from build123d import *

# Parameters (mm, degrees)
SKETCH1_R               = 20.450000000000003
BOSS_EXTRUDE1_DEPTH     = 15.875
CUT_EXTRUDE2_START      = -11.875
CUT_EXTRUDE2_DEPTH      = 11.875
M4_CLEARANCE_HOLE1_D    = 4.5
CHAMFER1_SIZE           = 4.7625
SHELL1_OUTLINE_R        = 20.45
SHELL1_DEPTH            = 10.284072775
SHELL1_2_DEPTH          = 2
BOSS_EXTRUDE2_START     = 2
BOSS_EXTRUDE2_DEPTH     = 2
CUT_EXTRUDE5_DEPTH      = 0.5
CUT_EXTRUDE7_DEPTH      = 42.774640932046694
CUT_EXTRUDE7_DEPTH_BACK = 42.774640932046694


with BuildPart() as part:
    # Sketch1 → Boss-Extrude1 (new body)
    # profile 1 of 2: a face of its own
    with BuildSketch(Plane.XY):
        with BuildLine():
            ThreePointArc((-4.449768205772106, -27.620494530122933), (-6.26579346059064, -23.208178662106004), (-9.919608253272203, -20.139609532026952))
            ThreePointArc((-9.919608253272203, -20.139609532026952), (-22.449999999999612, -2.260939e-11), (-9.919608253272486, 20.139609531981904))
            ThreePointArc((-9.919608253272486, 20.139609531981904), (-6.265793460590954, 23.208178662061), (-4.449768205772483, 27.620494530077963))
            ThreePointArc((-4.449768205772483, 27.620494530077963), (1.6339e-13, 31.449999999977553), (4.449768205772869, 27.620494530078034))
            ThreePointArc((4.449768205772869, 27.620494530078034), (6.265793460591407, 23.2081786620611), (9.919608253272981, 20.139609531982046))
            ThreePointArc((9.919608253272981, 20.139609531982046), (22.4500000000004, -2.229809e-11), (9.919608253273257, -20.13960953202682))
            ThreePointArc((9.919608253273257, -20.13960953202682), (6.265793460591725, -23.20817866210592), (4.449768205773249, -27.620494530122876))
            ThreePointArc((4.449768205773249, -27.620494530122876), (5.9636e-13, -31.450000000022463), (-4.449768205772106, -27.620494530122933))
        make_face()
        Circle(SKETCH1_R, mode=Mode.SUBTRACT)
    # profile 2 of 2: a face of its own
    with BuildSketch(Plane.XY):
        Circle(SKETCH1_R)
    extrude(amount=BOSS_EXTRUDE1_DEPTH)

    # Sketch3 → Cut-Extrude2 (cut)
    with BuildSketch(Plane.XY.offset(15.875).offset(CUT_EXTRUDE2_START)):
        with BuildLine():
            ThreePointArc((-9.919608253272486, 20.139609531981908), (2.3162e-13, 22.449999999977553), (9.919608253272981, 20.13960953198205))
            ThreePointArc((9.91960825327298, 20.139609531982046), (6.2657934605914, 23.208178662061094), (4.4497682057728625, 27.620494530078037))
            ThreePointArc((4.4497682057728625, 27.620494530078037), (1.6065e-13, 31.449999999977546), (-4.449768205772477, 27.620494530077963))
            ThreePointArc((-4.449768205772479, 27.620494530077963), (-6.265793460590951, 23.208178662061), (-9.919608253272482, 20.139609531981904))
        make_face()
        with BuildLine():
            ThreePointArc((4.449768205773246, -27.62049453012288), (6.265793460591725, -23.20817866210592), (9.919608253273257, -20.13960953202682))
            ThreePointArc((9.919608253273244, -20.139609532026824), (5.4515e-13, -22.45000000002246), (-9.919608253272205, -20.139609532026956))
            ThreePointArc((-9.9196082532722, -20.139609532026952), (-6.265793460590633, -23.208178662106), (-4.449768205772095, -27.620494530122933))
            ThreePointArc((-4.4497682057720995, -27.620494530122933), (5.9608e-13, -31.450000000022456), (4.449768205773246, -27.62049453012288))
        make_face()
    extrude(amount=CUT_EXTRUDE2_DEPTH, mode=Mode.SUBTRACT)

    # M4 Clearance Hole1 (through all)
    with Locations(Plane.XY.offset(4)):
        with Locations((0, -26.95), (0, 26.95)):
            Hole(M4_CLEARANCE_HOLE1_D / 2)

    # Chamfer1
    chamfer1_edges = [part.edges().sort_by_distance(p)[0] for p in [
        (9.91960825327299, 20.139609531982046, 15.875),
    ]]
    chamfer(chamfer1_edges, length=CHAMFER1_SIZE)

    # Shell1: read off the stored shape, not the designer's step
    # Shell1 outline → Shell1 (cut)
    with BuildSketch(Plane.XY):
        Circle(SHELL1_OUTLINE_R)
    extrude(amount=SHELL1_DEPTH, mode=Mode.SUBTRACT)

    # Shell1 2 outline → Shell1 2 (cut)
    with BuildSketch(Plane.XY):
        with BuildLine():
            ThreePointArc((9.035901505, -18.345434963), (0, -20.45), (-9.035901505, -18.345434963))
            ThreePointArc((-9.035901505, -18.345434963), (-5.656595992, -20.826114024), (-3.336769132, -24.317800965))
            ThreePointArc((-3.336769132, -24.317800965), (0, -22.7), (3.336769132, -24.317800965))
            ThreePointArc((3.336769132, -24.317800965), (5.656595992, -20.826114024), (9.035901505, -18.345434963))
        make_face()
        with BuildLine():
            ThreePointArc((-3.336769132, 24.317800965), (-5.656595992, 20.826114024), (-9.035901505, 18.345434963))
            ThreePointArc((-9.035901505, 18.345434963), (0, 20.45), (9.035901505, 18.345434963))
            ThreePointArc((9.035901505, 18.345434963), (5.656595992, 20.826114024), (3.336769132, 24.317800965))
            ThreePointArc((3.336769132, 24.317800965), (0, 22.7), (-3.336769132, 24.317800965))
        make_face()
    extrude(amount=SHELL1_2_DEPTH, mode=Mode.SUBTRACT)

    # Shell1 3 outline → Shell1 3 (revolve, cut)
    with BuildSketch(Plane.XZ):
        Polygon((16.859072875, 13.875), (0, 13.875), (0, 10.284072775), (20.45, 10.284072775), align=None)
    revolve(axis=Axis((0, 0, 0), (0, 0, 1)), mode=Mode.SUBTRACT)

    # Sketch6 → Boss-Extrude2 (add)
    with BuildSketch(Plane(origin=(0, 0, 2), x_dir=(-1, 0, 0), z_dir=(0, 0, -1)).offset(BOSS_EXTRUDE2_START)):
        with BuildLine():
            ThreePointArc((9.035901504651038, -18.34543496347422), (5.656595991725949, -20.826114024149227), (3.3367691319005477, -24.3178009648972))
            ThreePointArc((3.3367691319005477, -24.3178009648972), (-5.6684e-13, -22.70000000000008), (-3.3367691319011485, -24.317800964898304))
            ThreePointArc((-3.3367691319011485, -24.317800964898304), (-5.656595991726578, -20.826114024149597), (-9.035901504652076, -18.345434963474087))
            ThreePointArc((-9.035901504652076, -18.345434963474087), (-5.3382e-13, -20.45000000002246), (9.035901504651038, -18.34543496347422))
        make_face()
        with BuildLine():
            ThreePointArc((-9.035901504651829, 18.345434963429298), (-5.65659599172108, 20.826114024110222), (-3.336769131894781, 24.31780096486728))
            ThreePointArc((-3.336769131894781, 24.31780096486728), (-2.2525e-13, 22.699999999977557), (3.336769131894348, 24.317800964867242))
            ThreePointArc((3.336769131894348, 24.317800964867242), (5.656595991720593, 20.826114024110154), (9.03590150465129, 18.345434963429177))
            ThreePointArc((9.03590150465129, 18.345434963429177), (-2.5229e-13, 20.449999999977546), (-9.035901504651829, 18.345434963429298))
        make_face()
    extrude(amount=-BOSS_EXTRUDE2_DEPTH)

    # Sketch7 → Cut-Extrude5 (cut)
    with BuildSketch(Plane.XY.offset(15.875)):
        Polygon((-2.381250000000002, 9.524999999999997), (-2.381250000000001, 2.3812500000000005), (2.3812499999999996, 2.3812500000000005), (2.3812499999999983, 9.524999999999997), align=None)
        Polygon((2.3812499999999996, 2.3812500000000005), (-2.3812500000000014, 2.3812500000000005), (-2.3812500000000005, -2.3812499999999996), (2.3812499999999996, -2.3812499999999996), align=None)
        Polygon((9.525, 2.3812500000000005), (2.3812499999999996, 2.3812500000000005), (2.381249999999999, -2.3812499999999996), (9.525, -2.3812499999999996), align=None)
        Polygon((-2.3812500000000014, 2.3812500000000005), (-9.525, 2.3812500000000005), (-9.525, -2.3812500000000005), (-2.3812500000000005, -2.38125), align=None)
        Polygon((2.3812499999999996, -2.3812499999999996), (-2.3812500000000005, -2.38125), (-2.3812499999999996, -9.525000000000004), (2.3812499999999996, -9.525000000000004), align=None)
    extrude(amount=-CUT_EXTRUDE5_DEPTH, mode=Mode.SUBTRACT)

    # Sketch9 → Cut-Extrude7 (cut, two sides: drawn at the far end of the back side and taken through both)
    # profile 1 of 3: a face of its own
    with BuildSketch(Plane(origin=(0, 0, 0), x_dir=(0, 0, -1), z_dir=(1, 0, 0)).offset(-CUT_EXTRUDE7_DEPTH_BACK)):
        Polygon((-1.5018000000013485, 9.688999997177131), (-1.5018000000013485, -9.68900000282286), (-7.676800000001349, -9.689000002822862), (-7.676800000001349, 9.688999997177131), align=None)
        Polygon((-3.0018000000013485, 8.188999997177131), (-6.176800000001349, 8.188999997177124), (-6.176800000001349, -8.189000002822862), (-3.0018000000013485, -8.189000002822862), align=None, mode=Mode.SUBTRACT)
    # profile 2 of 3: a face of its own
    with BuildSketch(Plane(origin=(0, 0, 0), x_dir=(0, 0, -1), z_dir=(1, 0, 0)).offset(-CUT_EXTRUDE7_DEPTH_BACK)):
        Polygon((0, -9.68900000282286), (-1.5018000000013485, -9.68900000282286), (-1.5018000000013485, 9.688999997177131), (0, 9.68899999717713), align=None)
    # profile 3 of 3: a face of its own
    with BuildSketch(Plane(origin=(0, 0, 0), x_dir=(0, 0, -1), z_dir=(1, 0, 0)).offset(-CUT_EXTRUDE7_DEPTH_BACK)):
        Polygon((-3.0018000000013485, 8.188999997177131), (-3.0018000000013485, -8.189000002822862), (-6.176800000001349, -8.189000002822862), (-6.176800000001349, 8.188999997177124), align=None)
    extrude(amount=CUT_EXTRUDE7_DEPTH + CUT_EXTRUDE7_DEPTH_BACK, mode=Mode.SUBTRACT)


solid = part.part
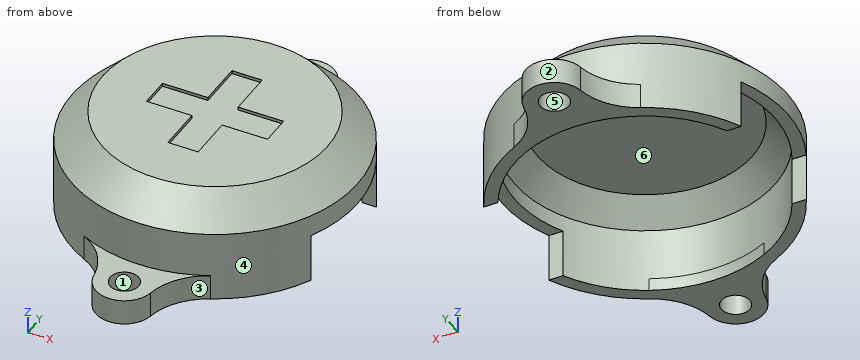
Source: CAD feature listing. Evaluate the final solid. Frame: model axes, mm. Face numbers are marked on the shaded views. A direction names the side the tool comes from. Give positions to 0.01 mm unless a question says otherwise; leave off trailing zeros. Write each loop counter-clockwise with the first axis right and the second up, starting at its lowest first coordinate (ties: lowest second). Pieces come first, ordered by that corner, then holes. Notation, with made-up numbers: M 63.5,85.5 L 109.5,85.5 A13 ccw 109.5,94.5 Z; hole C -9.5,47.25 d1. An arc over 180 degrees is marked long. Return JSON: item names as keys, results as strings. Group by question number.
1) Cut plane D-D, the plane y = 26.95. Output: boundary loops of the cut face in (x, z).
2) Cut plane B-B, the plane z = 6.75. Output: boundary loops of the cut face in (x, y), plus the area to 3 significant figures.
3) Pin query (flat end, axial travel): P1, Ø1.5, axis at x = 11, z = 8, coming from the +Y side; P2, Ø0.6, axis at x = -1, z = 15.5, coming from the +Y side; P3, Ø2, axis at x = 21, y = 4.5, coming from the -Z side. Return the tip coordinate at first contact, or that it passes through.
4) Pull-direction query (Y, two-part tool) for the marked faces 1, 2 and 3; classes: pulls with the +Y half, pulls with the -Y half, needs draft (parallel to the pull), parting line crosses it, or undercut.
5) Material intervals for line 1 along Y through (x, z) = (0, 1.6); line 2 along X through (y, z) = (0, 8.25), sorted ascending. Write a range as [from, to].
6) Set-up query: the marked faces 4, 5 and 6. Return all of +Z, -Z, +X, -X, +Y, -Y with unobstructed straight access to the full face (end or side cutting, diameter ignored); none if empty.
7) Cut plane A-A, the plane x = 0. Give the number of separate pieces and of enclosed holes in the cut face, plus the area to 3 significant figures.
Recorded:
{
 "1": {"outline": "M -4.57,0 L -2.25,0 L -2.25,4 L -4.57,4 Z; M 2.25,0 L 4.57,0 L 4.57,4 L 2.25,4 Z"},
 "2": {"outline": "M -20.25,-9.69 A22.45 ccw 20.25,-9.69 L 18.01,-9.69 A20.45 cw -18.01,-9.69 Z; M -20.25,9.69 L -18.01,9.69 A20.45 cw 18.01,9.69 L 20.25,9.69 A22.45 ccw Z", "area": "189 mm²"},
 "3": {"P1": "stops at y = 19.97", "P2": "stops at y = 18.34", "P3": "stops at z = 7.68"},
 "4": {"face 1": "undercut", "face 2": "pulls with the +Y half", "face 3": "pulls with the -Y half"},
 "5": {"line 1": "y = [-31.45, -29.2], [-24.7, -20.45], [20.45, 24.7], [29.2, 31.45]", "line 2": "x = [-22.45, -20.45], [20.45, 22.45]"},
 "6": {"face 4": "+Z", "face 5": "+Z, -Z", "face 6": "-Z"},
 "7": {"separate pieces": "3", "enclosed holes": "0", "area": "162 mm²"}
}
